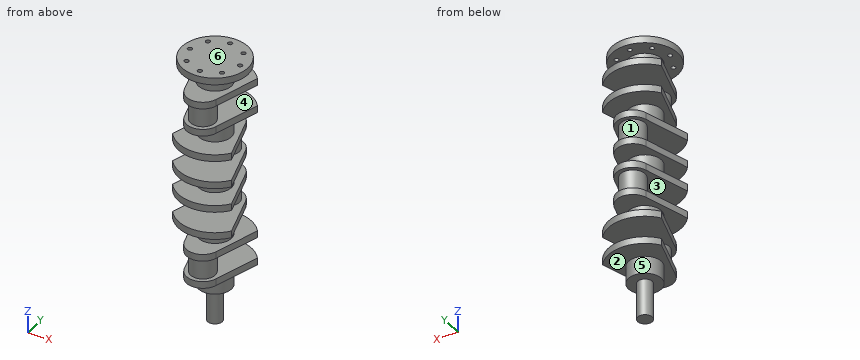
from build123d import *

# Parameters (mm, degrees)
BOSS_EXTRUDE1_DEPTH   = 15
SKETCH3_R             = 36
BOSS_EXTRUDE2_DEPTH   = 38
SKETCH4_R             = 27
BOSS_EXTRUDE3_DEPTH   = 46
BODY_MOVE_COPY3_ANGLE = 180
SKETCH5_R             = 16
BOSS_EXTRUDE4_DEPTH   = 80
SKETCH6_R             = 72
SKETCH6_R_2           = 5
BOSS_EXTRUDE5_DEPTH   = 15


with BuildPart() as part:
    # Sketch2 → Boss-Extrude1 (new body)
    with BuildSketch(Plane.XY):
        with BuildLine():
            Line((-64.569893475, 47.23059238), (-34.517510455, -54.224552409))
            ThreePointArc((-34.517510455, -54.224552409), (0, -80), (34.517510455, -54.224552409))
            Line((34.517510455, -54.224552409), (64.569893475, 47.23059238))
            ThreePointArc((64.569893475, 47.23059238), (0, 80), (-64.569893475, 47.23059238))
        make_face()
    boss_extrude1 = extrude(amount=BOSS_EXTRUDE1_DEPTH)

    # Sketch3 → Boss-Extrude2 (add)
    with BuildSketch(Plane.XY.offset(15)):
        Circle(SKETCH3_R)
    boss_extrude2 = extrude(amount=BOSS_EXTRUDE2_DEPTH)

    # Sketch4 → Boss-Extrude3 (add)
    with BuildSketch(Plane(origin=(0, 0, 0), x_dir=(-1, 0, 0), z_dir=(0, 0, -1))):
        with Locations((0, -44)):
            Circle(SKETCH4_R)
    extrude(amount=BOSS_EXTRUDE3_DEPTH)

    # Mirror2: Boss-Extrude1, Boss-Extrude2 across plane
    add(boss_extrude1.mirror(Plane(origin=(0, 0, -23), x_dir=(1, 0, 0), z_dir=(0, 0, -1))))
    add(boss_extrude2.mirror(Plane(origin=(0, 0, -23), x_dir=(1, 0, 0), z_dir=(0, 0, -1))))


with BuildPart() as body_2:
    # Mirror6: mirrored copy
    add(part.part.mirror(Plane(origin=(0, 0, -80), x_dir=(1, 0, 0), z_dir=(0, 0, -1))))


with BuildPart() as part_1:
    # Body-Move/Copy3: moved
    add(part.part.rotate(Axis((0, 0, 0), (0, 0, 1)), BODY_MOVE_COPY3_ANGLE))


with BuildPart() as body_3:
    # Mirror7: mirrored copy
    add(body_2.part.mirror(Plane.XY.offset(34)))

    # Sketch6 → Boss-Extrude5 (add)
    with BuildSketch(Plane.XY.offset(281)):
        Circle(SKETCH6_R)
        with Locations((0, 55)):
            Circle(SKETCH6_R_2, mode=Mode.SUBTRACT)
        with Locations((38.890872965, 38.890872965)):
            Circle(SKETCH6_R_2, mode=Mode.SUBTRACT)
        with Locations((55, 0)):
            Circle(SKETCH6_R_2, mode=Mode.SUBTRACT)
        with Locations((38.890872965, -38.890872965)):
            Circle(SKETCH6_R_2, mode=Mode.SUBTRACT)
        with Locations((0, -55)):
            Circle(SKETCH6_R_2, mode=Mode.SUBTRACT)
        with Locations((-38.890872965, -38.890872965)):
            Circle(SKETCH6_R_2, mode=Mode.SUBTRACT)
        with Locations((-55, 0)):
            Circle(SKETCH6_R_2, mode=Mode.SUBTRACT)
        with Locations((-38.890872965, 38.890872965)):
            Circle(SKETCH6_R_2, mode=Mode.SUBTRACT)
    extrude(amount=BOSS_EXTRUDE5_DEPTH)


with BuildPart() as body_4:
    # Mirror7 2: mirrored copy
    add(part_1.part.mirror(Plane.XY.offset(34)))


with BuildPart() as body_2_1:
    add(body_2.part)

    # Sketch5 → Boss-Extrude4 (add)
    with BuildSketch(Plane(origin=(0, 0, -213), x_dir=(-1, 0, 0), z_dir=(0, 0, -1))):
        Circle(SKETCH5_R)
    extrude(amount=BOSS_EXTRUDE4_DEPTH)


with BuildPart() as body_3_1:
    add(body_3.part)

    # Combine1: union body 4, part, body 2
    add(body_4.part)
    add(part_1.part)
    add(body_2_1.part)


solid = body_3_1.part
Model file for the job. Use its own axes, mm. Face numbers are marked on the shaded views. A direction names the side the tool comes from. Round coordinates to 2 decimals unless told otherwise and drop trailing zeros. Loops run counter-clockwise (first coordinate to the right, second up) from the corner with the lowest first, then second, coordinate; pieces in that order, holes last. Notation, with made-up numbers: M 34,50.5 L 60,50.5 A21 cw 60,58.5 Z; hole C 86,40.25 d9. An arc over 180 degrees is marked long. One line per question, with ' | ' between items.
1) Drill centre lines: line 1 along Z through (x, y) = (-38, -54.5); line 2 along Z through (x, y) = (10, 1); line 3 along Y through (x, z) = (0, 290). Where is each one in solid material? Low to high.
Solved:
line 1: z = -61 to -46, 0 to 15, 53 to 68, 114 to 129, 281 to 296 | line 2: z = -293 to -160, -114 to -46, 0 to 68, 114 to 182, 228 to 296 | line 3: y = -72 to -60, -50 to 50, 60 to 72
2) Mould opens along Z. For the marked faces 3, 4, 5 and 6 say: +Z half, -Z half, draft (parallel to the pull), parting line (faces both ways), or undercut.
Solved:
face 3: undercut | face 4: undercut | face 5: draft | face 6: +Z half
3) 3-axis set-ups, long thin cutter, end or side, ignore diameter. For the marked faces 1 and 2: which of +Z, -Z, +X, -X, +Y, -Y reach the whole face in a straight line?
Solved:
face 1: none | face 2: -Z
4) Band-saw the part on B-B (z = -125.5). Give the cut face in (x, y).
Solved:
outline: C 0,-44 d54
5) Band-saw the part on A-A (z = -206). Give the cut face in (x, y).
Solved:
outline: C 0,0 d72
6) Flat gauge pins, fed straight in: pin 1 (12 mm diameter, centred on x = 56.5, y = 31.5, fed in from -Z); pin 2 (2 mm diameter, centred on y = -11.5, z = 236.5, fed in from +X); pin 3 (10 mm diameter, centred on x = -16.5, y = 30, fed in from -Z). Where does each tip first touch, or does it go through?
Solved:
pin 1: stops at z = -175 | pin 2: stops at x = 47.47 | pin 3: stops at z = -213
